```python
from build123d import *

# Parameters (mm, degrees)
SKETCH_1_W          = 24
SKETCH_1_H          = 12.5
EXTRUDE_1_DEPTH     = 9
SKETCH_2_W          = 24
SKETCH_2_H          = 8.2
CUT_EXTRUDE_1_DEPTH = 6.2
SKETCH_3_R          = 0.5
CUT_EXTRUDE_2_DEPTH = 17.25
SKETCH_4_R          = 0.6
CUT_EXTRUDE_3_DEPTH = 17.25
SKETCH_5_R          = 1
CUT_EXTRUDE_4_DEPTH = 7
CHAMFER_1_SIZE      = 1


with BuildPart() as part:
    # 草图1 → 凸台-拉伸1 (new body)
    with BuildSketch(Plane(origin=(0, 0, 0), x_dir=(1, 0, 0), z_dir=(0, 1, 0))):
        Rectangle(SKETCH_1_W, SKETCH_1_H)
    extrude(amount=EXTRUDE_1_DEPTH)

    # 草图2 → 切除-拉伸1 (cut)
    with BuildSketch(Plane.XZ):
        Rectangle(SKETCH_2_W, SKETCH_2_H)
    extrude(amount=-CUT_EXTRUDE_1_DEPTH, mode=Mode.SUBTRACT)

    # 草图3 → 切除-拉伸2 (cut, through all)
    with BuildSketch(Plane(origin=(0, 9, 0), x_dir=(1, 0, 0), z_dir=(0, 1, 0))):
        with Locations(Location((-8.5, 5.125, 0), (0, 0, 270))):
            Circle(SKETCH_3_R)
        with Locations(Location((8.5, 5.125, 0), (0, 0, 90))):
            Circle(SKETCH_3_R)
        with Locations(Location((8.5, -5.125, 0), (0, 0, 270))):
            Circle(SKETCH_3_R)
        with Locations(Location((-8.5, -5.125, 0), (0, 0, 90))):
            Circle(SKETCH_3_R)
    extrude(amount=-CUT_EXTRUDE_2_DEPTH, mode=Mode.SUBTRACT)

    # 草图4 → 切除-拉伸3 (cut, through all)
    with BuildSketch(Plane(origin=(0, 9, 0), x_dir=(1, 0, 0), z_dir=(0, 1, 0))):
        with Locations(Location((-8.5, -0.25, 0), (0, 0, 270))):
            Circle(SKETCH_4_R)
        with Locations(Location((8.5, -0.25, 0), (0, 0, 90))):
            Circle(SKETCH_4_R)
    extrude(amount=-CUT_EXTRUDE_3_DEPTH, mode=Mode.SUBTRACT)

    # 草图5 → 切除-拉伸4 (cut)
    with BuildSketch(Plane(origin=(0, 9, 0), x_dir=(1, 0, 0), z_dir=(0, 1, 0))):
        with Locations(Location((-8.5, 5.125, 0), (0, 0, 270))):
            Circle(SKETCH_5_R)
        with Locations(Location((8.5, 5.125, 0), (0, 0, 270))):
            Circle(SKETCH_5_R)
        with Locations(Location((-8.5, -5.125, 0), (0, 0, 270))):
            Circle(SKETCH_5_R)
        with Locations(Location((8.5, -5.125, 0), (0, 0, 270))):
            Circle(SKETCH_5_R)
    extrude(amount=-CUT_EXTRUDE_4_DEPTH, mode=Mode.SUBTRACT)

    # 倒角1
    # the kernel refuses this chamfer: 1 mm, written as the material it takes off along each edge
    with BuildSketch(Plane(origin=(-14.571682988, 9, -6.25), x_dir=(0, 0.027495876610585623, 0.9996219169112968), z_dir=(1, 0, 0))) as chamfer_1_piece_1:
        Polygon((CHAMFER_1_SIZE * 0.999621916911, CHAMFER_1_SIZE * 0.0274958766106), (-CHAMFER_1_SIZE * 0.0274958766106, CHAMFER_1_SIZE * 0.999621916911), (0, 0), align=None)
    extrude(amount=29.143365976, mode=Mode.SUBTRACT)
    with BuildSketch(Plane(origin=(14.571682988, 9, 6.25), x_dir=(0, -0.9996219169112968, 0.027495876610586487), z_dir=(-1, 0, 0))) as chamfer_1_piece_2:
        Polygon((CHAMFER_1_SIZE * 0.999621916911, -CHAMFER_1_SIZE * 0.0274958766106), (-CHAMFER_1_SIZE * 0.0274958766106, -CHAMFER_1_SIZE * 0.999621916911), (0, 0), align=None)
    extrude(amount=29.143365976, mode=Mode.SUBTRACT)


solid = part.part
```
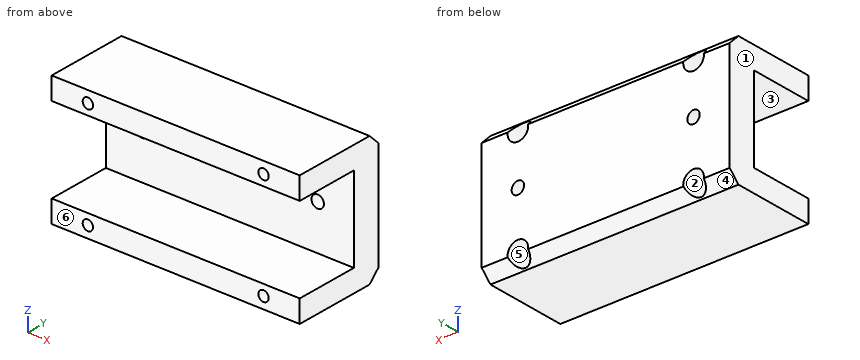
Verification items for the finished model (mm, model axes). Face numbers are marked on the shaded views. A direction names the side the tool comes from. Coordinates: 2 decimals unless noted, no trailing zeros. Write each loop counter-clockwise with the first axis right and the second up, starting at its lowest first coordinate (ties: lowest second). Pieces come first, ordered by that corner, then holes. Notation, with made-up numbers: M 23.5,86 L 49.5,86 A16 cw 49.5,105 Z; hole C 16.5,-22 d6. An arc over 180 degrees is marked long. One line per item, written item: value.
Item 1: Section check A-A, the plane y = 4. Record the boundary of the cut face in (x, z) (3 decimals), plus the area to 3 significant figures.
Check sheet entries:
outline: M -12,-6.25 L 12,-6.25 L 12,-4.1 L -12,-4.1 Z; M -12,4.1 L 12,4.1 L 12,6.25 L -12,6.25 Z; hole C -8.5,-5.125 d2; hole C -8.5,5.125 d2; hole C 8.5,-5.125 d2; hole C 8.5,5.125 d2
area: 90.6 mm^2
Item 2: Mould release check, pull along Z, two halves, no side actions. Record for the marked faces 4, 5 and 6: pulls with the +Z half, pulls with the -Z half, needs draft (parallel to the pull), parting line crosses it, or undercut.
Check sheet entries:
face 4: pulls with the -Z half
face 5: undercut
face 6: needs draft
Item 3: Gauge pin test, flat ends, axial feed: pin 1 Ø1 at (x, z) = (9, -5.5) entering from +Y; pin 2 Ø1.9 at (x, z) = (8.5, 0.25) entering from -Y; pin 3 Ø1.1 at (x, z) = (-8.5, 0.25) entering from +Y; pin 4 Ø1.8 at (x, z) = (8.5, 5.125) entering from +Y. Record the tip position at first contact, or that the pin passes through.
Check sheet entries:
pin 1: stops at y = 8.9
pin 2: stops at y = 6.2
pin 3: passes through
pin 4: stops at y = 2
Item 4: Scan lines: line 1 along Z through (x, y) = (5.5, 2.75); line 2 along X through (y, z) = (7.55, 0.25); line 3 along Z through (x, y) = (-8.25, 6.5). Record each from-to range of solid material in increasing order.
Check sheet entries:
line 1: z = -6.25 to -4.1, 4.1 to 6.25
line 2: x = -12 to -9.1, -7.9 to 7.9, 9.1 to 12
line 3: z = -6.25 to -6.09, -4.16 to -0.3, 0.8 to 4.16, 6.09 to 6.25
Item 5: Section check B-B, the plane z = 0.25. Record the boundary of the cut face in (x, y).
Check sheet entries:
outline: M -12,6.2 L -9.1,6.2 L -9.1,9 L -12,9 Z; M -7.9,6.2 L 7.9,6.2 L 7.9,9 L -7.9,9 Z; M 9.1,6.2 L 12,6.2 L 12,9 L 9.1,9 Z
Item 6: Section check C-C, the plane x = -3.5. Record the boundary of the cut face in (y, z).
Check sheet entries:
outline: M 0,-6.25 L 8,-6.25 L 9,-5.25 L 9,5.25 L 8,6.25 L 0,6.25 L 0,4.1 L 6.2,4.1 L 6.2,-4.1 L 0,-4.1 Z
Item 7: Section check D-D, the plane x = -8.5. Record the boundary of the cut face in (y, z) (3 decimals), plus the area to 3 significant figures.
Check sheet entries:
outline: M 0,-6.25 L 8,-6.25 L 8.125,-6.125 L 2,-6.125 L 2,-5.625 L 0,-5.625 Z; M 0,-4.625 L 2,-4.625 L 2,-4.125 L 9,-4.125 L 9,-0.35 L 6.2,-0.35 L 6.2,-4.1 L 0,-4.1 Z; M 0,4.1 L 6.2,4.1 L 6.2,0.85 L 9,0.85 L 9,4.125 L 2,4.125 L 2,4.625 L 0,4.625 Z; M 0,5.625 L 2,5.625 L 2,6.125 L 8.125,6.125 L 8,6.25 L 0,6.25 Z
area: 26.1 mm^2
Item 8: Access from +Z, -Z, +X, -X, +Y, -Y to the whole of each face (thin tool, end or side, straight path). Record for the marked faces 1, 2 and 3.
Check sheet entries:
face 1: +Z, -Z, -X, +Y, -Y
face 2: +Y
face 3: +X, -X, -Y
